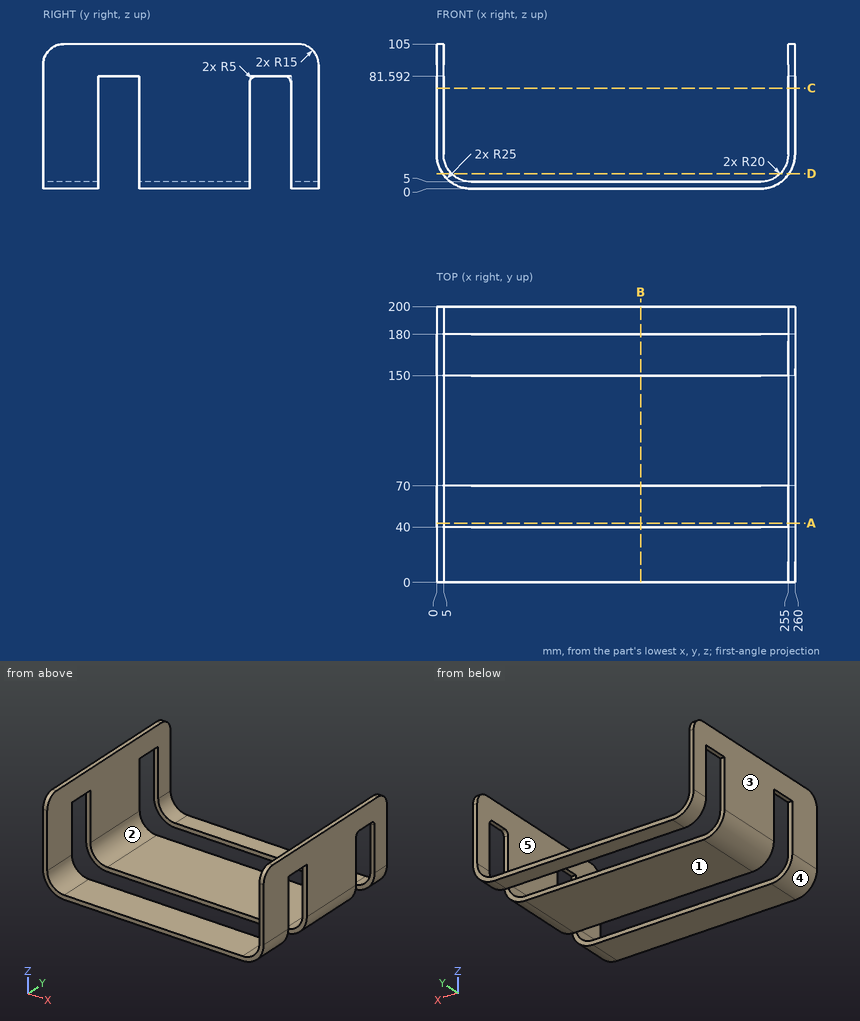
Study the drawing (mm; zero at the part's minimum x, y, z) and answer. A direction names the side the tool comes from. Give positions to 0.01 mm unless a question says otherwise; leave off trailing zeros. Loops run counter-clockwise (first coordinate to the right, second up) from the corner with the lowest first, then second, coordinate; pieces in that order, holes last. Notation, with made-up numbers: (77, -28) - (82, -28) arc R9 cw to (82, -24) - close; hole circle Ø5 at (-11.5, 80.5). An arc over 180 degrees is marked (long way). One line per question, with ' | ' between items.
(1) The part is cut by section B-B (x = 148). Write down the section's boundary in (y, z), then the cut area to 3 significant figures.
Recorded:
outline: (0, 0) - (40, 0) - (40, 5) - (0, 5) - close; (70, 0) - (150, 0) - (150, 5) - (70, 5) - close; (180, 0) - (200, 0) - (200, 5) - (180, 5) - close | area: 700 mm²
(2) The part is cut by section A-A (y = 43). Write down the section's boundary in (x, z), then the cut area to 3 significant figures.
Recorded:
outline: (0, 81.59) - (5, 81.59) - (5, 105) - (0, 105) - close; (255, 81.59) - (260, 81.59) - (260, 105) - (255, 105) - close | area: 234 mm²
(3) Each of these flat-tipped pins is pushed along its axis until it touches: pin 1 Ø1.5 at (x, y) = (257.5, 169.5) entering from -Z; pin 2 Ø6 at (x, y) = (211.5, 108) entering from +Z. Where does it stop, or does it pass through?
Recorded:
pin 1: stops at z = 81.59 | pin 2: stops at z = 5
(4) Straight lines are drawn through the part: probe 1 along X at (y, z) = (35.5, 35); probe 2 along Z at (x, y) = (52.5, 23.5); probe 3 along X at (y, z) = (32.5, 8) (1 decimal). For each, find the intervals that lie inside material, in ascending order.
Recorded:
probe 1: x = 0 to 5, 255 to 260 | probe 2: z = 0 to 5 | probe 3: x = 6.7 to 14.5, 245.5 to 253.3
(5) The part is cut by section D-D (z = 11). Write down the section's boundary in (x, y).
Recorded:
outline: (4.29, 0) - (10.72, 0) - (10.72, 40) - (4.29, 40) - close; (4.29, 70) - (10.72, 70) - (10.72, 150) - (4.29, 150) - close; (4.29, 180) - (10.72, 180) - (10.72, 200) - (4.29, 200) - close; (249.28, 0) - (255.71, 0) - (255.71, 40) - (249.28, 40) - close; (249.28, 70) - (255.71, 70) - (255.71, 150) - (249.28, 150) - close; (249.28, 180) - (255.71, 180) - (255.71, 200) - (249.28, 200) - close
(6) The part is cut by section C-C (z = 73). Write down the section's boundary in (x, y).
Recorded:
outline: (0, 0) - (5, 0) - (5, 40) - (0, 40) - close; (0, 70) - (5, 70) - (5, 150) - (0, 150) - close; (0, 180) - (5, 180) - (5, 200) - (0, 200) - close; (255, 0) - (260, 0) - (260, 40) - (255, 40) - close; (255, 70) - (260, 70) - (260, 150) - (255, 150) - close; (255, 180) - (260, 180) - (260, 200) - (255, 200) - close
(7) The mould has two halves that part along X. Classify the marked faces 1, 2 and 3: +X half, -X half, draft (parallel to the pull), parting line (faces both ways), or undercut.
Recorded:
face 1: draft | face 2: undercut | face 3: -X half
(8) A tool of negligible diameter and unlimited length cuts with its end or side. For the marked faces 4 and 5, from which of +Z, -Z, +X, -X, +Y, -Y can it reach the whole face along a straight path? Write none if from no direction.
Recorded:
face 4: -Z, -X, +Y, -Y | face 5: +Z, +Y, -Y
